Could you check a few things on this model? Use its own coordinates, in mm. Face numbers are marked on the shaded views. A direction names the side the tool comes from. Give positions to 0.01 mm unless a question says otherwise; leave off trailing zeros. Order: outer loops, then holes, each group sorted by start corner. A loop starts at its lowest first (then second) coordinate and runs counter-clockwise, first axis right, second up.
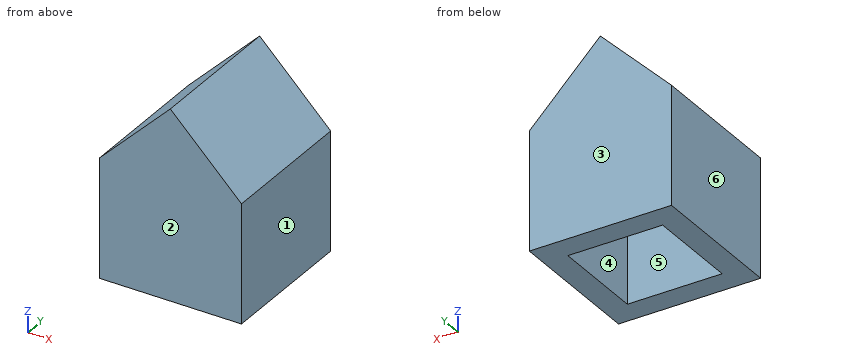
from build123d import *

# Parameters (mm, degrees)
F0_W        = 30
F0_H        = 30
F0_W_2      = 20
F0_H_2      = 20
F1_DEPTH    = 25
F2_W        = 30
F2_H        = 30
F3_DEPTH    = 25
F4_T1_DEPTH = 158.5841493983


# Not quite as in the source:
# - a fillet or chamfer that OpenCascade refuses, or shapes differently, is made with other operations: its cross-section is extruded or revolved along the edge and cut away or added


with BuildPart() as f1:
    # F0 (on Top) → F1 (new body)
    with BuildSketch(Plane.XY):
        with Locations((15, 15)):
            Rectangle(F0_W, F0_H)
        with Locations((15, 15)):
            Rectangle(F0_W_2, F0_H_2, mode=Mode.SUBTRACT)
    extrude(amount=F1_DEPTH)

    # F2 (on face) → F3 (join)
    with BuildSketch(Plane.XY.offset(25)):
        with Locations((15, 15)):
            Rectangle(F2_W, F2_H)
    extrude(amount=F3_DEPTH)

    # F4: chamfer of 25 on 2 edges, made by hand

    # F4_s2 → F4_t1 (cut)
    with BuildSketch(Plane.XZ.offset(-94.2920746991)):
        Polygon((0, 25), (25, 50), (0, 50), align=None)
        Polygon((5, 50), (30, 25), (30, 50), align=None)
    extrude(amount=F4_T1_DEPTH, mode=Mode.SUBTRACT)


solid = f1.part
Item 1: Imagine slicing it at C-C on x = 10.5. List the corners of the cut face in (y, z) for me, then the cut area to 3 significant figures.
Findings:
outline: (0, 0) - (5, 0) - (5, 25) - (25, 25) - (25, 0) - (30, 0) - (30, 35.5) - (0, 35.5) - close
area: 565 mm2
Item 2: We'd pull the mould along Y, two halves only. Please class the marked faces 1, 2, 3 and 4: +Y half, -Y half, draft (parallel to the pull), parting line (faces both ways), or undercut.
Findings:
face 1: draft
face 2: -Y half
face 3: +Y half
face 4: undercut
Item 3: For the marked faces 5 and 6, which set-ups out of +Z, -Z, +X, -X, +Y, -Y let a thin tool reach every point of the face, with its end or its side?
Findings:
face 5: -Z
face 6: +Z, -Z, -X, +Y, -Y
Item 4: For pin 1 (10 mm diameter, centred on x = 23.5, y = 9.5, fed in from +Z); pin 2 (5 mm diameter, centred on y = 5.5, z = 31.5, fed in from +X); pin 3 (16 mm diameter, centred on x = 16.5, y = 15.5, fed in from -Z), each with a flat end and sliding along its axis, tell me the tip position at first contact or that it passes through.
Findings:
pin 1: stops at z = 36.5
pin 2: stops at x = 26
pin 3: stops at z = 25
Item 5: Please list where these lines run through material, in increasing order: line 1 along Y through (x, z) = (7.5, 10.5); line 2 along Z through (x, y) = (27, 19).
Findings:
line 1: y = 0 to 5, 25 to 30
line 2: z = 0 to 28
Item 6: Imagine slicing it at D-D on z = 27. List the corners of the cut face in (x, y) for me, then the cut area to 3 significant figures.
Findings:
outline: (2, 0) - (28, 0) - (28, 30) - (2, 30) - close
area: 780 mm2
Item 7: Imagine slicing it at B-B on z = 18.5. List the corners of the cut face in (x, y) for me.
Findings:
outline: (0, 0) - (30, 0) - (30, 30) - (0, 30) - close; hole (5, 5) - (25, 5) - (25, 25) - (5, 25) - close
Item 8: Imagine slicing it at A-A on y = 23. List the corners of the cut face in (x, z) for me, then the cut area to 3 significant figures.
Findings:
outline: (0, 0) - (5, 0) - (5, 25) - (25, 25) - (25, 0) - (30, 0) - (30, 25) - (15, 40) - (0, 25) - close
area: 475 mm2
